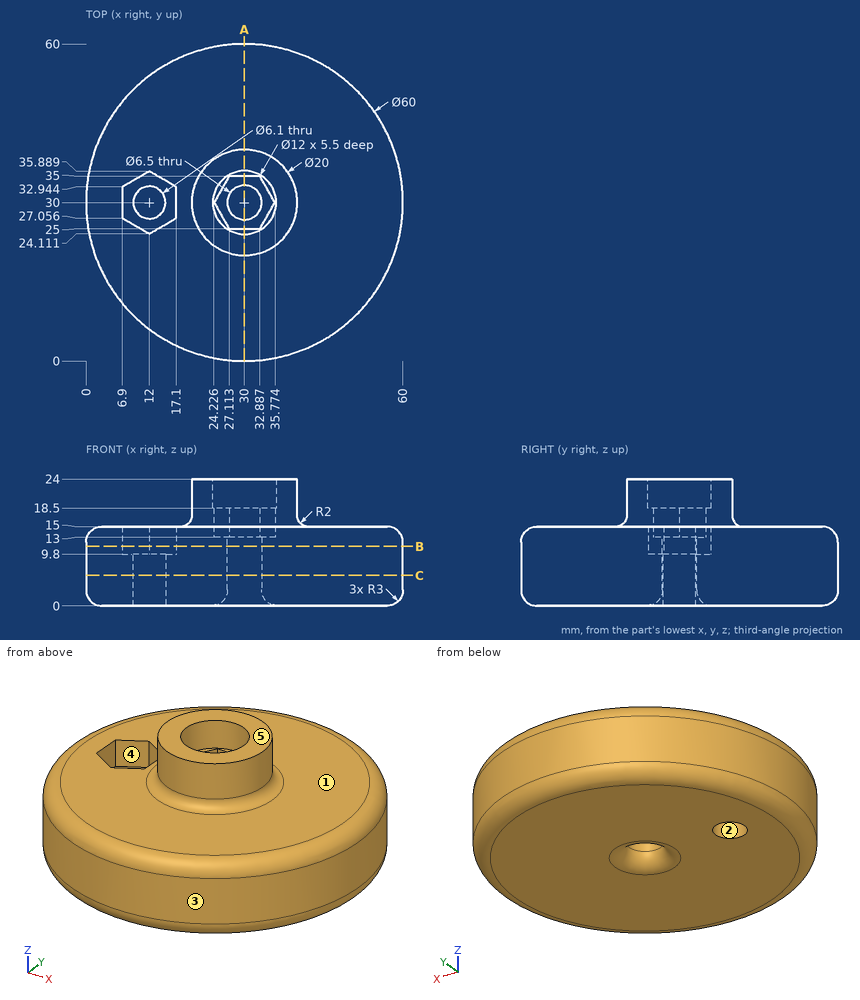
Print and shaded views of the part. All mm, measured from the part's lowest x, y and z. A direction names the side the tool comes from. Coordinates: 2 decimals unless noted, no trailing zeros. Loops run counter-clockwise (first coordinate to the right, second up) from the corner with the lowest first, then second, coordinate; pieces in that order, holes last. Notation, with made-up numbers: (8, 1) -> (45, 1) arc R19 ccw to (45, 29) -> close; hole circle Ø5 at (59, -12.75). An arc over 180 degrees is marked (long way). Use a Markdown table: item, result. Add a question column.
Item 1: Flat gauge pins, fed straight in: P1, Ø4.5, axis at x = 29.5, z = 17, coming from the +Y side (1 decimal); P2, Ø1, axis at x = 38, z = 4, coming from the -Y side; P3, Ø3, axis at x = 31, y = 32, coming from the +Z side. Where does each tip first touch, or does it go through?
Item 2: Probe probe 1 along Y at (x, z) = (30, 10.75); probe 2 along X at (y, z) = (28, 6) (1 decimal); probe 3 along Z at (x, y) = (47, 21). List the from-to ranges inside material, lowest first.
Item 3: Which spindle directions (+Z, -Z, +X, -X, +Y, -Y) get a long thin tool onto all of the face, cutting with end or side? Do the marked faces 4 and 5. Say none if no direction does.
Item 4: Band-saw the part on B-B on z = 11.25. Give the number of separate pieces and of enclosed holes in the cut face, plus the area to 3 significant figures.
Item 5: Band-saw the part on C-C on z = 5.75. Write the cut outline in (x, y).
Item 6: Pull direction Y, two halves, no side cores. Call the marked faces 1, 2 and 3: +Y half, -Y half, draft (parallel to the pull), parting line (faces both ways), or undercut.
Item 7: Band-saw the part on A-A on x = 30. Write the cut outline in (y, z).
Geometry says:
| question | item | result |
|---|---|---|
| 1 | P1 | y = 58.2 |
| 1 | P2 | y = 0.95 |
| 1 | P3 | z = 13 |
| 2 | probe 1 | 0 to 26.75, 33.25 to 60 |
| 2 | probe 2 | 0.1 to 9.7, 14.3 to 27.4, 32.6 to 59.9 |
| 2 | probe 3 | 0 to 15 |
| 3 | face 4 | +Z |
| 3 | face 5 | +Z, +X, -X, +Y, -Y |
| 4 | separate pieces | 1 |
| 4 | enclosed holes | 2 |
| 4 | area | 2,700 mm² |
| 5 | outline | circle Ø60 at (30, 30); hole circle Ø6.1 at (12, 30); hole circle Ø6.5 at (30, 30) |
| 6 | face 1 | draft |
| 6 | face 2 | undercut |
| 6 | face 3 | parting line |
| 7 | outline | (0, 3) arc R3 ccw to (3, 0) -> (23.75, 0) arc R3 ccw to (26.75, 3) -> (26.75, 13) -> (25, 13) -> (25, 18.5) -> (24, 18.5) -> (24, 24) -> (20, 24) -> (20, 17) arc R2 cw to (18, 15) -> (3, 15) arc R3 ccw to (0, 12) -> close; (33.25, 3) arc R3 ccw to (36.25, 0) -> (57, 0) arc R3 ccw to (60, 3) -> (60, 12) arc R3 ccw to (57, 15) -> (42, 15) arc R2 cw to (40, 17) -> (40, 24) -> (36, 24) -> (36, 18.5) -> (35, 18.5) -> (35, 13) -> (33.25, 13) -> close |
